from build123d import *

# Parameters (mm, degrees)
EXTRUDE_1_DEPTH     = 245
SKETCH_2_R          = 5
CUT_EXTRUDE_1_DEPTH = 10
SKETCH_3_R          = 5
CUT_EXTRUDE_2_DEPTH = 10


with BuildPart() as part:
    # Эскиз1 → Вытянуть-Тонкостенный1 (new body)
    with BuildSketch(Plane(origin=(0, 0, 0), x_dir=(1, 0, 0), z_dir=(0, 1, 0))):
        Polygon((0, 65), (0, 0), (65, 0), (65, 4), (4, 4), (4, 65), align=None)
    extrude(amount=EXTRUDE_1_DEPTH)

    # Эскиз2 → Вырез-Вытянуть1 (cut)
    with BuildSketch(Plane.XY):
        with Locations((31, 225)):
            Circle(SKETCH_2_R)
        with Locations((31, 125)):
            Circle(SKETCH_2_R)
        with Locations((31, 25)):
            Circle(SKETCH_2_R)
    extrude(amount=-CUT_EXTRUDE_1_DEPTH, mode=Mode.SUBTRACT)

    # Эскиз3 → Вырез-Вытянуть2 (cut)
    with BuildSketch(Plane.ZY):
        with Locations((-31, 225)):
            Circle(SKETCH_3_R)
        with Locations((-31, 125)):
            Circle(SKETCH_3_R)
        with Locations((-31, 25)):
            Circle(SKETCH_3_R)
    extrude(amount=-CUT_EXTRUDE_2_DEPTH, mode=Mode.SUBTRACT)


solid = part.part
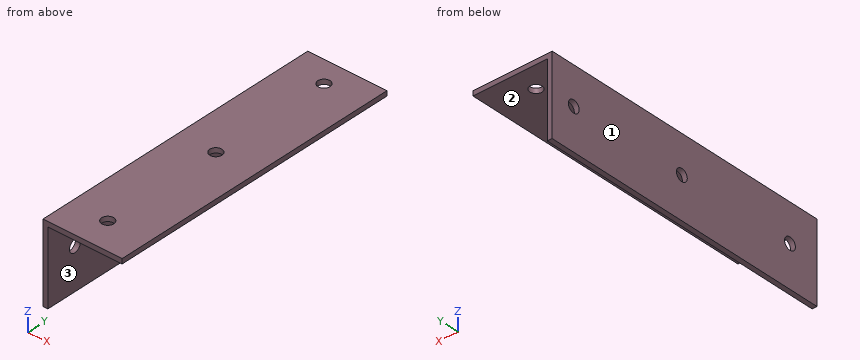
For this review, take the finished solid that the model builds, in its own axes (mm). Face numbers are marked on the shaded views. Give positions to 0.01 mm unless a question says otherwise; leave off trailing zeros. Order: outer loops, then holes, each group sorted by start corner. A loop starts at its lowest first (then second) coordinate and runs counter-clockwise, first axis right, second up. Notation, with made-up numbers: (-14, -17) -> (5, -17) arc R31 cw to (5, 19) -> close; hole circle Ø5 at (-12.75, 0). An arc over 180 degrees is marked (long way). Write item = value, one per line.
1) We need section C-C, the plane y = 25. Give the boundary of the cut face in (x, z), and give its area (3 significant figures).
Findings:
outline = (0, -65) -> (4, -65) -> (4, -36) -> (0, -36) -> close; (0, -26) -> (4, -26) -> (4, -4) -> (26, -4) -> (26, 0) -> (0, 0) -> close; (36, -4) -> (65, -4) -> (65, 0) -> (36, 0) -> close
area = 424 mm^2
2) To check wall thickness, follow L1, parallel to Y at x = 31, z = -2.05; L2, parallel to Z at x = 7.5, y = 95; L3, parallel to X at y = 206.5, z = -22. State the ranges of each line that lie inside material, in increasing order. Write a range as from..to.
Findings:
L1 = 0..20, 30..120, 130..220, 230..245
L2 = -4..0
L3 = 0..4
3) We need section A-A, the plane x = 31. Give the boundary of the cut face in (y, z), and give its area (3 significant figures).
Findings:
outline = (0, -4) -> (20, -4) -> (20, 0) -> (0, 0) -> close; (30, -4) -> (120, -4) -> (120, 0) -> (30, 0) -> close; (130, -4) -> (220, -4) -> (220, 0) -> (130, 0) -> close; (230, -4) -> (245, -4) -> (245, 0) -> (230, 0) -> close
area = 860 mm^2
4) Insertion check: pin 1 (18.5 mm diameter, centred on x = 48.5, y = 65, fed in from -Z); pin 2 (13 mm diameter, centred on y = 125, z = -31, fed in from +X); pin 3 (6 mm diameter, centred on x = 31, y = 225, fed in from -Z). Each pin has a flat end and moves straight along its axis. Give the tip position at first contact, or say it passes through.
Findings:
pin_1 = -4
pin_2 = 4
pin_3 = through
5) Draft analysis for pull direction X (two halves, no side actions). For the marked faces 1, 2 and 3, state which applies: pulls with the +X half, pulls with the -X half, needs draft (parallel to the pull), parting line crosses it, or undercut.
Findings:
face_1 = pulls with the -X half
face_2 = needs draft
face_3 = pulls with the +X half
6) We need section B-B, the plane z = -31. Give the boundary of the cut face in (x, y).
Findings:
outline = (0, 0) -> (4, 0) -> (4, 20) -> (0, 20) -> close; (0, 30) -> (4, 30) -> (4, 120) -> (0, 120) -> close; (0, 130) -> (4, 130) -> (4, 220) -> (0, 220) -> close; (0, 230) -> (4, 230) -> (4, 245) -> (0, 245) -> close
7) We need section D-D, the plane y = 145. Give the boundary of the cut face in (x, z), and give its area (3 significant figures).
Findings:
outline = (0, -65) -> (4, -65) -> (4, -4) -> (65, -4) -> (65, 0) -> (0, 0) -> close
area = 504 mm^2
